```python
from build123d import *

# Parameters (mm, degrees)
F0_R         = 3.2512
F1_DEPTH     = 10.0076
F2_R         = 36.4998
F3_DEPTH     = 1.6002
F4_R         = 7.9375
F5_DEPTH     = 31.75
F6_SIZE      = 0.381
F7_R         = 12.7
F7_R_2       = 7.9375
F8_DEPTH     = 1.6002
F10_DEPTH    = 140.9954
F11_T1_DEPTH = 156.8704
F12_R        = 1.6002
F13_R        = 4.826
F14_DEPTH    = 12.7
F14_TAPER    = 1


# Not quite as in the source:
# - a fillet or chamfer that OpenCascade refuses, or shapes differently, is made with other operations: its cross-section is extruded or revolved along the edge and cut away or added


with BuildPart() as f1:
    # F0 (on Front) → F1 (new body)
    with BuildSketch(Plane.XZ):
        with BuildLine():
            ThreePointArc((42.926, 36.576), (41.0661280605, 41.0661280605), (36.576, 42.926))
            Line((36.576, 42.926), (-36.576, 42.926))
            ThreePointArc((-36.576, 42.926), (-41.0661280605, 41.0661280605), (-42.926, 36.576))
            Line((-42.926, 36.576), (-42.926, -36.576))
            ThreePointArc((-42.926, -36.576), (-41.0661280605, -41.0661280605), (-36.576, -42.926))
            Line((-36.576, -42.926), (36.576, -42.926))
            ThreePointArc((36.576, -42.926), (41.0661280605, -41.0661280605), (42.926, -36.576))
            Line((42.926, -36.576), (42.926, 36.576))
        make_face()
        with Locations((-34.925, -34.925)):
            Circle(F0_R, mode=Mode.SUBTRACT)
        with Locations((34.925, -34.925)):
            Circle(F0_R, mode=Mode.SUBTRACT)
        with Locations((-34.925, 34.925)):
            Circle(F0_R, mode=Mode.SUBTRACT)
        with Locations((34.925, 34.925)):
            Circle(F0_R, mode=Mode.SUBTRACT)
    extrude(amount=-F1_DEPTH)

    # F2 (on Front) → F3 (join)
    with BuildSketch(Plane.XZ):
        Circle(F2_R)
    extrude(amount=F3_DEPTH)

    # F4 (on Front) → F5 (join)
    with BuildSketch(Plane.XZ):
        Circle(F4_R)
    extrude(amount=F5_DEPTH)

    # F6
    f6_edges = [f1.edges().sort_by_distance(p)[0] for p in [
        (-7.9375, -31.75, 0),
    ]]
    chamfer(f6_edges, length=F6_SIZE)

    # F7 (on face) → F8 (cut)
    with BuildSketch(Plane.XZ.offset(1.6002)):
        Circle(F7_R)
        Circle(F7_R_2, mode=Mode.SUBTRACT)
    extrude(amount=-F8_DEPTH, mode=Mode.SUBTRACT)

    # F9 (on face) → F10 (join)
    with BuildSketch(Plane(origin=(0, 10.0076, 0), x_dir=(-1, 0, 0), z_dir=(0, 1, 0))):
        with BuildLine():
            ThreePointArc((-26.7554344057, 34.925), (-29.1482447689, 29.1482447689), (-34.925, 26.7554344057))
            Line((-34.925, 26.7554344057), (-42.926, 26.7554344057))
            Line((-42.926, 26.7554344057), (-42.926, -26.7554344057))
            Line((-42.926, -26.7554344057), (-34.925, -26.7554344057))
            ThreePointArc((-34.925, -26.7554344057), (-29.1482447689, -29.1482447689), (-26.7554344057, -34.925))
            Line((-26.7554344057, -34.925), (-26.7554344057, -42.926))
            Line((-26.7554344057, -42.926), (26.7554344057, -42.926))
            Line((26.7554344057, -42.926), (26.7554344057, -34.925))
            ThreePointArc((26.7554344057, -34.925), (29.1482447689, -29.1482447689), (34.925, -26.7554344057))
            Line((34.925, -26.7554344057), (42.926, -26.7554344057))
            Line((42.926, -26.7554344057), (42.926, 26.7554344057))
            Line((42.926, 26.7554344057), (34.925, 26.7554344057))
            ThreePointArc((34.925, 26.7554344057), (29.1482447689, 29.1482447689), (26.7554344057, 34.925))
            Line((26.7554344057, 34.925), (26.7554344057, 42.926))
            Line((26.7554344057, 42.926), (-26.7554344057, 42.926))
            Line((-26.7554344057, 42.926), (-26.7554344057, 34.925))
        make_face()
    extrude(amount=F10_DEPTH)

    # F11: fillet of radius 6.35 on 8 edges, made by hand

    # F11_s2 → F11_t1 (cut)
    with BuildSketch(Plane.XZ.offset(-166.878)):
        with BuildLine():
            ThreePointArc((20.4054344057, 42.926), (24.8955624662, 41.0661280605), (26.7554344057, 36.576))
            Line((26.7554344057, 36.576), (26.7554344057, 42.926))
            Line((26.7554344057, 42.926), (20.4054344057, 42.926))
        make_face()
        with BuildLine():
            ThreePointArc((42.926, 20.4054344057), (41.0661280605, 24.8955624662), (36.576, 26.7554344057))
            Line((36.576, 26.7554344057), (42.926, 26.7554344057))
            Line((42.926, 26.7554344057), (42.926, 20.4054344057))
        make_face()
        with BuildLine():
            ThreePointArc((42.926, -20.4054344057), (41.0661280605, -24.8955624662), (36.576, -26.7554344057))
            Line((36.576, -26.7554344057), (42.926, -26.7554344057))
            Line((42.926, -26.7554344057), (42.926, -20.4054344057))
        make_face()
        with BuildLine():
            ThreePointArc((20.4054344057, -42.926), (24.8955624662, -41.0661280605), (26.7554344057, -36.576))
            Line((26.7554344057, -36.576), (26.7554344057, -42.926))
            Line((26.7554344057, -42.926), (20.4054344057, -42.926))
        make_face()
        with BuildLine():
            ThreePointArc((-20.4054344057, 42.926), (-24.8955624662, 41.0661280605), (-26.7554344057, 36.576))
            Line((-26.7554344057, 36.576), (-26.7554344057, 42.926))
            Line((-26.7554344057, 42.926), (-20.4054344057, 42.926))
        make_face()
        with BuildLine():
            ThreePointArc((-42.926, 20.4054344057), (-41.0661280605, 24.8955624662), (-36.576, 26.7554344057))
            Line((-36.576, 26.7554344057), (-42.926, 26.7554344057))
            Line((-42.926, 26.7554344057), (-42.926, 20.4054344057))
        make_face()
        with BuildLine():
            ThreePointArc((-42.926, -20.4054344057), (-41.0661280605, -24.8955624662), (-36.576, -26.7554344057))
            Line((-36.576, -26.7554344057), (-42.926, -26.7554344057))
            Line((-42.926, -26.7554344057), (-42.926, -20.4054344057))
        make_face()
        with BuildLine():
            ThreePointArc((-20.4054344057, -42.926), (-24.8955624662, -41.0661280605), (-26.7554344057, -36.576))
            Line((-26.7554344057, -36.576), (-26.7554344057, -42.926))
            Line((-26.7554344057, -42.926), (-20.4054344057, -42.926))
        make_face()
    extrude(amount=F11_T1_DEPTH, mode=Mode.SUBTRACT)

    # F12
    f12_edges = [f1.edges().sort_by_distance(p)[0] for p in [
        (24.895562, 151.003, 41.066128),
    ]]
    fillet(f12_edges, radius=F12_R)

    # F13 (on face) → F14 (join)
    with BuildSketch(Plane(origin=(0, 0, -42.926), x_dir=(1, 0, 0), z_dir=(0, 0, -1))):
        with Locations((0, -136.7028)):
            Circle(F13_R)
    extrude(amount=F14_DEPTH, taper=F14_TAPER)


solid = f1.part
```
CAD build for the part. Positions are in the model's coordinates, mm. A direction names the side the tool comes from. Round coordinates to 2 decimals unless told otherwise and drop trailing zeros. Write each loop counter-clockwise with the first axis right and the second up, starting at its lowest first coordinate (ties: lowest second). Pieces come first, ordered by that corner, then holes. Notation, with made-up numbers: (34.5, 48) - (80.5, 48) arc R30 cw to (80.5, 84) - close; hole circle Ø9 at (51, 33.25). An arc over 180 degrees is marked (long way). Write item = value, one per line. Start each with the question number.
Q1. Mould opens along Z. For faces 5 (the flat face through (16, -1.6, 1)), 6 (the cylindrical face through (-38.173, 4.934, -34.782)), 7 (the cylindrical face through (41.115, 80.681, 24.846)) say: pulls with the +Z half, pulls with the -Z half, needs draft (parallel to the pull), parting line crosses it, or undercut.
Q2. Band-saw the part on A-A (y = 6). Give the cut face in (x, z) (3 decimals).
Q3. Band-saw the part on B-B (z = 0). Give the cut face in (x, y).
Q4. Which spindle directions (+Z, -Z, +X, -X, +Y, -Y) get a long thin tool onto all of the face, cutting with end or side? Do faces 1 (the cylindrical face through (41.115, 80.681, -24.846)), 2 (the cylindrical face through (-41.115, 80.681, -24.846)), 3 (the cylindrical face through (-41.115, 80.681, 24.846)), 4 (the cylindrical face through (-28.965, -0.789, -22.21)). Say none if no direction does.
Q5. Band-saw the part on D-D (z = 16). Give the cut face in (x, y), then the cut area to 3 significant figures.
Q6. Band-saw the part on C-C (x = -17). Give the cut face in (y, z), then the cut area to 3 significant figures.
Q7. Drop flat-ended pins along their axis: pin 1 (8 mm diameter, centred on x = 7, z = -27, fed in from -Y); pin 2 (7.5 mm diameter, centred on x = -34.925, z = 34.925, fed in from +Y); pin 3 (0.8 mm diameter, centred on x = 36, y = 94.5, fed in from -Z). Give the stop position or say it passes through.
Q8. Probe L1, parallel to Z at x = 0, y = -1.25; L2, parallel to Y at x = 7.5, z = -36.5; L3, parallel to Z at x = 35.5, y = 50.5. List the from-to ranges inside material, lowest first. Write a range as from..to.
Answers below:
q1.face_5 = needs draft
q1.face_6 = undercut
q1.face_7 = pulls with the +Z half
q2.outline = (-42.926, -36.576) arc R6.35 ccw to (-36.576, -42.926) - (36.576, -42.926) arc R6.35 ccw to (42.926, -36.576) - (42.926, 36.576) arc R6.35 ccw to (36.576, 42.926) - (-36.576, 42.926) arc R6.35 ccw to (-42.926, 36.576) - close; hole circle Ø6.502 at (-34.925, -34.925); hole circle Ø6.502 at (-34.925, 34.925); hole circle Ø6.502 at (34.925, -34.925); hole circle Ø6.502 at (34.925, 34.925)
q3.outline = (-42.93, 0) - (-36.5, 0) - (-36.5, -1.6) - (-12.7, -1.6) - (-12.7, 0) - (-7.94, 0) - (-7.94, -31.37) - (-7.56, -31.75) - (7.56, -31.75) - (7.94, -31.37) - (7.94, 0) - (12.7, 0) - (12.7, -1.6) - (36.5, -1.6) - (36.5, 0) - (42.93, 0) - (42.93, 149.4) arc R1.6 ccw to (41.33, 151) - (-41.33, 151) arc R1.6 ccw to (-42.93, 149.4) - close
q4.face_1 = -Z, +X, +Y
q4.face_2 = -Z, -X, +Y
q4.face_3 = +Z, -X, +Y
q4.face_4 = -Y
q5.outline = (-42.93, 0) - (-32.81, 0) - (-32.81, -1.6) - (32.81, -1.6) - (32.81, 0) - (42.93, 0) - (42.93, 149.4) arc R1.6 ccw to (41.33, 151) - (-41.33, 151) arc R1.6 ccw to (-42.93, 149.4) - close
q5.area = 13,100 mm2
q6.outline = (-1.6, -32.3) - (0, -32.3) - (0, -42.93) - (149.4, -42.93) arc R1.6 ccw to (151, -41.33) - (151, 41.33) arc R1.6 ccw to (149.4, 42.93) - (0, 42.93) - (0, 32.3) - (-1.6, 32.3) - close
q6.area = 13,100 mm2
q7.pin_1 = -1.6
q7.pin_2 = 10.01
q7.pin_3 = -26.76
q8.L1 = -36.5..-12.7, -7.94..7.94, 12.7..36.5
q8.L2 = 0..151
q8.L3 = -26.76..26.76
